from build123d import *

# Parameters (mm, degrees)
F0_R     = 3
F1_DEPTH = 150
F2_W     = 52
F2_H     = 30
F3_DEPTH = 3
F5_DEPTH = 2


with BuildPart() as f1:
    # F0 (on Top) → F1 (new body)
    with BuildSketch(Plane.XY):
        Circle(F0_R)
    extrude(amount=F1_DEPTH)

    # F2 (on Front) → F3 (join, symmetric)
    with BuildSketch(Plane.XZ):
        with Locations((27.0199, 135)):
            Rectangle(F2_W, F2_H)
    extrude(amount=F3_DEPTH, both=True)

    # F4 (on face) → F5 (cut)
    with BuildSketch(Plane.XZ.offset(3)):
        Polygon((11.0199, 120), (53.0199, 120), (53.0199, 150), (11.0199, 150), (13.0199, 148.321801), (11.0199, 146.666667), (13.0199, 144.988467), (11.0199, 143.333333), (13.0199, 141.655134), (11.0199, 140), (13.0199, 138.321801), (11.0199, 136.666667), (13.0199, 134.988467), (11.0199, 133.333333), (13.0199, 131.655134), (11.0199, 130), (13.0199, 128.321801), (11.0199, 126.666667), (13.0199, 124.988467), (11.0199, 123.333333), (13.0199, 121.655134), align=None)
    extrude(amount=-F5_DEPTH, mode=Mode.SUBTRACT)


solid = f1.part
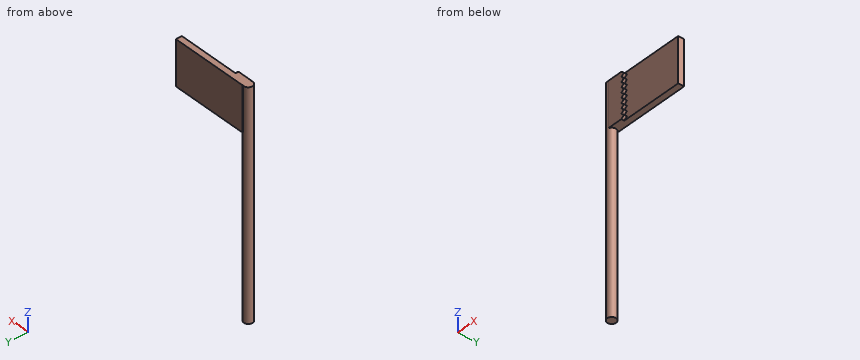
CAD build for the part. Positions are in the model's coordinates, mm. Round coordinates to 2 decimals unless told otherwise and drop trailing zeros. Loops run counter-clockwise (first coordinate to the right, second up) from the corner with the lowest first, then second, coordinate; pieces in that order, holes last.
(1) Cut at A-A (y = -1.9). Give the cut face in (x, z), plus the area to 3 significant figures.
(2) Cut at C-C (x = 29.5). Give the cut face in (y, z), plus the area to 3 significant figures.
(3) Wall check: line 1 along Z through (x, y) = (38.5, 0.35); line 2 along X through (y, z) = (-1, 110); line 3 along X through (y, z) = (0.3, 42). Give the ranges that are in metal, low to high.
(4) Cut at B-B (z = 57). Give the cut face in (x, y), plus the area to 3 significant figures.
(5) Drop flat-ended pins along their axis: pin 1 (2 mm diameter, centred on x = 4.5, y = 1.5, fed in from -Z); pin 2 (15 mm diameter, centred on x = 34.5, z = 137, fed in from -Y). Give the stop position or say it passes through.
Findings below:
1. outline: (-2.32, 0) - (2.32, 0) - (2.32, 120) - (11.02, 120) - (13.02, 121.66) - (11.02, 123.33) - (13.02, 124.99) - (11.02, 126.67) - (13.02, 128.32) - (11.02, 130) - (13.02, 131.66) - (11.02, 133.33) - (13.02, 134.99) - (11.02, 136.67) - (13.02, 138.32) - (11.02, 140) - (13.02, 141.66) - (11.02, 143.33) - (13.02, 144.99) - (11.02, 146.67) - (13.02, 148.32) - (11.02, 150) - (-2.32, 150) - close
1. area: 987 mm2
2. outline: (-1, 120) - (3, 120) - (3, 150) - (-1, 150) - close
2. area: 120 mm2
3. line 1: z = 120 to 150
3. line 2: x = -2.83 to 2.83
3. line 3: x = -2.98 to 2.98
4. outline: circle Ø6 at (0, 0)
4. area: 28.3 mm2
5. pin 1: stops at z = 120
5. pin 2: stops at y = -1
